Autodesk Inventor part; units mm, degrees
ref_plane "YZ Plane" through (0, 0, 0) normal (1, 0, 0) x (0, 1, 0)
ref_plane "XZ Plane" through (0, 0, 0) normal (0, 1, 0) x (-1, 0, 0)
ref_plane "XY Plane" through (0, 0, 0) normal (0, 0, 1) x (1, 0, 0)
sketch "スケッチ1" plane through (0, 0, 0) normal (0, 0, 1) x (1, 0, 0)
  line L0 (-50, 0) -> (50, 0) construction
  circle A0 centre (-50, 0) radius 4.05
  circle A1 centre (50, 0) radius 4.05
  line L1 (-50, 8.5) -> (50, 8.5)
  line L2 (-50, -8.5) -> (50, -8.5)
  arc A2 (-50, 8.5) -> (-50, -8.5) centre (-50, 0) ccw
  arc A3 (50, -8.5) -> (50, 8.5) centre (50, 0) ccw
  line L3 (55.697, 6.3082) -> (35, 25)
  line L4 (35, 25) -> (-10, 25)
  line L5 (-10, 25) -> (-24.9014, 8.5)
  line L6 (-16.3218, 18) -> (42.751, 18) construction
  line L7 (-10, 25) -> (-10, 18) construction
  line L8 (35, 25) -> (35, 18) construction
  circle A4 centre (32.5, 21.5) radius 1.55
  circle A5 centre (-7.5, 21.5) radius 1.55
  circle A6 centre (12.5, 21.5) radius 1.55
  line L9 (-10, 21.5) -> (35, 21.5) construction
  line L10 (35, 24) -> (-10, 24) construction
  line L11 (-10, 24) -> (-10, 19) construction
  line L12 (-10, 19) -> (35, 19) construction
  line L13 (35, 19) -> (35, 24) construction
  point P0 (0, 0)
  point P1 (0, 0)
  dimension "d0" = 100
  dimension "d1" = 8.1
  dimension "d2" = 8.5
  dimension "d8" = 8.1
  dimension "d10" = 7
  dimension "d11" = 45
  dimension "d12" = 2.5
  dimension "d13" = 3.1
  dimension "d14" = 2.5
  dimension "d15" = 15
  dimension "d17" = 5
  dimension "d18" = 19
extrude "押し出し1" add sketch "スケッチ1" along normal blind 2
fillet "フィレット1" radius 5 3 edges at (-24.9014, 8.5, 1) (-10, 25, 1) (35, 25, 1)
sketch "スケッチ2" plane through (0, 0, 2) normal (0, 0, 1) x (1, 0, 0)
  arc A0 (50, -8.5) -> (55.697, 6.3082) centre (50, 0) ccw
  line L0 (18, -20) -> (-35.4549, -20) construction
  line L1 (-76.9607, -11.5) -> (-72, -11.5)
  line L2 (-72, -11.5) -> (-62, -7)
  line L3 (-62, -7) -> (-32, -7)
  line L4 (-32, -7) -> (-22, -11.5)
  line L5 (-22, -11.5) -> (-17.0393, -11.5)
  line L6 (-17.0393, -11.5) -> (-17.0393, -12.4)
  line L7 (-17.0393, -12.4) -> (-76.9607, -12.4)
  line L8 (-76.9607, -12.4) -> (-76.9607, -11.5)
  line L9 (-31.9893, -6.95) -> (-62.0107, -6.95)
  line L10 (-62.0107, -6.95) -> (-72.0107, -11.45)
  line L11 (-72.0107, -11.45) -> (-77.0107, -11.45)
  line L12 (-77.0107, -11.45) -> (-77.0107, -12.45)
  line L13 (-77.0107, -12.45) -> (-16.9893, -12.45)
  line L14 (-16.9893, -12.45) -> (-16.9893, -11.45)
  line L15 (-16.9893, -11.45) -> (-21.9893, -11.45)
  line L16 (-21.9893, -11.45) -> (-31.9893, -6.95)
  circle A1 centre (-50, 0) radius 4.05
  circle A2 centre (-50, 0) radius 5.5 construction
  circle A3 centre (50, 0) radius 4.05
  line L17 (83.3205, -17.7128) -> (50, 0) construction
  line L18 (50, 0) -> (18, -20) construction
  line L19 (83.3205, -17.7128) -> (37.8533, -17.7128) construction
  line L20 (-11.6402, -10.1128) -> (48.2812, -10.1128)
  line L21 (48.2812, -10.1128) -> (48.2812, -9.2128)
  line L22 (48.2812, -9.2128) -> (43.3205, -9.2128)
  line L23 (43.3205, -9.2128) -> (33.3205, -4.7128)
  line L24 (33.3205, -4.7128) -> (3.3205, -4.7128)
  line L25 (3.3205, -4.7128) -> (-6.6795, -9.2128)
  line L26 (-6.6795, -9.2128) -> (-11.6402, -9.2128)
  line L27 (-11.6402, -9.2128) -> (-11.6402, -10.1128)
  line L28 (-6.6902, -9.1628) -> (3.3098, -4.6628)
  line L29 (3.3098, -4.6628) -> (33.3312, -4.6628)
  line L30 (33.3312, -4.6628) -> (43.3312, -9.1628)
  line L31 (43.3312, -9.1628) -> (48.3312, -9.1628)
  line L32 (48.3312, -9.1628) -> (48.3312, -10.1628)
  line L33 (48.3312, -10.1628) -> (-11.6902, -10.1628)
  line L34 (-11.6902, -10.1628) -> (-11.6902, -9.1628)
  line L35 (-11.6902, -9.1628) -> (-6.6902, -9.1628)
  point P0 (0, 0)
  dimension "d19" = 20
  dimension "d20" = 32
  dimension "d21" = 40
  dimension "d22" = 10
  dimension "d23" = 8.5
  dimension "d24" = 10
  dimension "d25" = 30
  dimension "d26" = 13
  dimension "d27" = 0.05
  dimension "d32" = 11
  dimension "d33" = 120
  dimension "d34" = 1
  dimension "d36" = 5
  dimension "d37" = 40
  dimension "d38" = 8.5
  dimension "d39" = 0.05
extrude "押し出し2" cut sketch "スケッチ2" against normal blind 10 contours L1 L2 L3 L4 L5 L6 L7 L8 | L16 L15 L14 L13 L12 L11 L10 L9 | L27 L26 L25 L24 L23 L22 L21 L20 | L28 L29 L30 L31 L32 L33 L34 L35
fillet "フィレット2" radius 2 7 edges at (-28.5448, -8.5, 1) (-31.9893, -6.95, 1) (-5.2173, -8.5, 1) (3.3098, -4.6628, 1) (41.8583, -8.5, 1) (33.3312, -4.6628, 1) (-54.8936, -6.95, 1)
sketch "スケッチ3" plane through (0, 0, 0) normal (0, 0, -1) x (-1, 0, 0)
  circle A0 centre (7.5, 21.5) radius 1.55
  circle A1 centre (7.5, 21.5) radius 1.55
  circle A2 centre (-12.5, 21.5) radius 1.55
  circle A3 centre (-12.5, 21.5) radius 1.55
  circle A4 centre (-32.5, 21.5) radius 1.55
  circle A5 centre (-32.5, 21.5) radius 1.55
  point P0 (0, 0)
extrude "押し出し3" add sketch "スケッチ3" against normal up to surface (2 mm away)
equation "\"d8\" = d1"
equation "\"d14\" = d12"
equation "\"d24\" = d22"
equation "\"d37\" = d21"
equation "\"d38\" = d23"
properties part number "rinnku" material "GFRP"
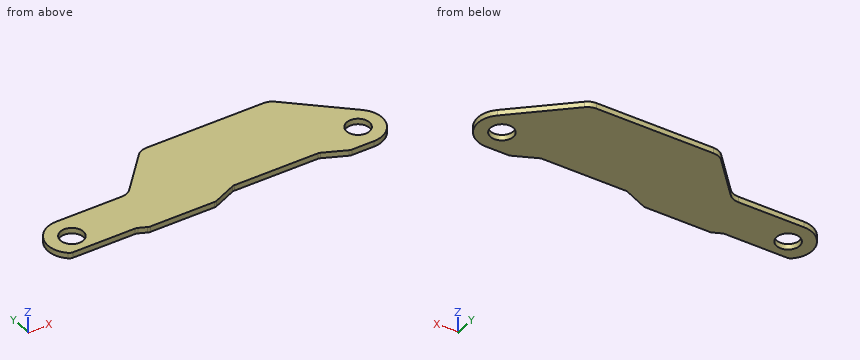
Verification items for the finished model (mm, model axes). Round coordinates to 2 decimals unless told otherwise and drop trailing zeros. Loops run counter-clockwise (first coordinate to the right, second up) from the corner with the lowest first, then second, coordinate; pieces in that order, holes last. Notation, with made-up numbers: (54, -31.5) - (103, -31.5) arc R18 ccw to (103, -12.5) - close; hole circle Ø5 at (35.5, -17). An arc over 180 degrees is marked (long way). Use a Markdown table: item, result. Add a question column.
1. Section check D-D, the plane y = 21. Record the boundary of the cut face in (x, z).
2. Gauge pin test, flat ends, axial feed: pin 1 (1 mm diameter, centred on x = -37.5, z = 1, fed in from +Y); pin 2 (0.6 mm diameter, centred on x = 15, z = 0.5, fed in from -Y); pin 3 (1 mm diameter, centred on y = 6, z = 0.5, fed in from -X); pin 4 (6.5 mm diameter, centred on x = 50, y = 0, fed in from -Z). Record the tip position at first contact, or that the pin passes through.
3. Section check A-A, the plane y = 0. Record the boundary of the cut face in (x, z).
4. Section check B-B, the plane z = 1.1. Record the boundary of the cut face in (x, y).
5. Section check C-C, the plane x = 26. Record the boundary of the cut face in (y, z), plus the area to 3 significant figures.
6. Thickness scan on probe 1 along Y at (x, z) = (-50, 1.65); probe 2 along Y at (x, z) = (28, 0.45); probe 3 along X at (y, z) = (-1, 1). Record the ranges inside material, lowest first. Write a range as [from, to].
Checks:
| question | item | result |
|---|---|---|
| 1 | outline | (-13.61, 0) - (39.43, 0) - (39.43, 2) - (-13.61, 2) - close |
| 2 | pin 1 | stops at y = 8.5 |
| 2 | pin 2 | stops at y = -4.66 |
| 2 | pin 3 | stops at x = -56.48 |
| 2 | pin 4 | passes through |
| 3 | outline | (-58.5, 0) - (-54.05, 0) - (-54.05, 2) - (-58.5, 2) - close; (-45.95, 0) - (45.95, 0) - (45.95, 2) - (-45.95, 2) - close; (54.05, 0) - (58.5, 0) - (58.5, 2) - (54.05, 2) - close |
| 4 | outline | (-55.51, -6.47) arc R2 ccw to (-54.21, -6.95) - (-32.42, -6.95) arc R2 cw to (-31.6, -7.13) - (-28.94, -8.32) arc R2 ccw to (-28.12, -8.5) - (-5.65, -8.5) arc R2 ccw to (-4.83, -8.32) - (2.92, -4.84) arc R2 cw to (3.74, -4.66) - (32.9, -4.66) arc R2 cw to (33.72, -4.84) - (41.47, -8.32) arc R2 ccw to (42.29, -8.5) - (50, -8.5) arc R8.5 ccw to (55.7, 6.31) - (36.43, 23.71) arc R5 ccw to (33.08, 25) - (-7.78, 25) arc R5 ccw to (-11.49, 23.35) - (-23.41, 10.15) arc R5 cw to (-27.12, 8.5) - (-50, 8.5) arc R8.5 ccw to start; hole circle Ø8.1 at (-50, 0); hole circle Ø8.1 at (50, 0) |
| 5 | outline | (-4.66, 0) - (25, 0) - (25, 2) - (-4.66, 2) - close |
| 5 | area | 59.3 mm^2 |
| 6 | probe 1 | y = [-6.95, -4.05], [4.05, 8.5] |
| 6 | probe 2 | y = [-4.66, 25] |
| 6 | probe 3 | x = [-58.44, -53.92], [-46.08, 46.08], [53.92, 58.44] |
